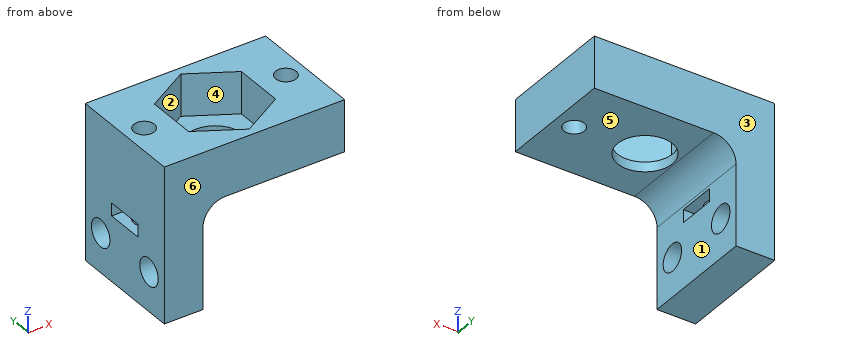
from build123d import *

# Parameters (mm, degrees)
BOSS_EXTRUDE1_DEPTH = 18
CUT_EXTRUDE1_DEPTH  = 6.5
SKETCH4_R           = 1.6
CUT_EXTRUDE2_DEPTH  = 17
SKETCH5_W           = 2
SKETCH5_H           = 6
CUT_EXTRUDE3_DEPTH  = 6
SKETCH6_R           = 4.25
CUT_EXTRUDE4_DEPTH  = 6
FILLET1_R           = 3.5
SKETCH7_R           = 2.1
CUT_EXTRUDE5_DEPTH  = 6


with BuildPart() as part:
    # Sketch1 → Boss-Extrude1 (new body)
    with BuildSketch(Plane(origin=(0, 0, 0), x_dir=(1, 0, 0), z_dir=(0, 1, 0))):
        Polygon((0, 24.076190476), (0, 0), (28, 0), (28, 8), (6, 8), (6, 24.076190476), align=None)
    extrude(amount=BOSS_EXTRUDE1_DEPTH)

    # Sketch3 → Cut-Extrude1 (cut)
    with BuildSketch(Plane.XY):
        Polygon((20.75, 5.102885683), (20.75, 12.897114317), (14, 16.794228634), (7.25, 12.897114317), (7.25, 5.102885683), (14, 1.205771366), align=None)
    extrude(amount=-CUT_EXTRUDE1_DEPTH, mode=Mode.SUBTRACT)

    # Sketch4 → Cut-Extrude2 (cut)
    with BuildSketch(Plane.XY):
        with Locations((25, 9)):
            Circle(SKETCH4_R)
        with Locations((3, 9)):
            Circle(SKETCH4_R)
    extrude(amount=-CUT_EXTRUDE2_DEPTH, mode=Mode.SUBTRACT)

    # Sketch5 → Cut-Extrude3 (cut)
    with BuildSketch(Plane.ZY):
        with Locations((-13, 9)):
            Rectangle(SKETCH5_W, SKETCH5_H)
    extrude(amount=-CUT_EXTRUDE3_DEPTH, mode=Mode.SUBTRACT)

    # Sketch6 → Cut-Extrude4 (cut)
    with BuildSketch(Plane.XY.offset(-6.5)):
        with Locations((14, 9)):
            Circle(SKETCH6_R)
    extrude(amount=-CUT_EXTRUDE4_DEPTH, mode=Mode.SUBTRACT)

    # Fillet1
    fillet1_edges = [part.edges().sort_by_distance(p)[0] for p in [
        (6, 9, -8),
    ]]
    fillet(fillet1_edges, radius=FILLET1_R)

    # Sketch7 → Cut-Extrude5 (cut)
    with BuildSketch(Plane(origin=(6, 0, 0), x_dir=(0, 0, -1), z_dir=(1, 0, 0))):
        with Locations((18, 14.5)):
            Circle(SKETCH7_R)
        with Locations(Location((18, 3.5, 0), (0, 0, 180))):
            Circle(SKETCH7_R)
    extrude(amount=-CUT_EXTRUDE5_DEPTH, mode=Mode.SUBTRACT)


solid = part.part
Build history of the part. All positions in model axes, mm. Face numbers are marked on the shaded views. A direction names the side the tool comes from. Coordinates: 2 decimals unless noted, no trailing zeros. Order: outer loops, then holes, each group sorted by start corner. A loop starts at its lowest first (then second) coordinate and runs counter-clockwise, first axis right, second up. Notation, with made-up numbers: (-37, 78) -> (-5, 78) arc R16 ccw to (-5, 108) -> close; hole circle Ø8 at (46, -35.75). An arc over 180 degrees is marked (long way). One line per item, written item: value.
(1) Slice it at C-C, the plane z = -13.5. List the corners of the cut face in (x, y), plus the area to 3 significant figures.
Checked values:
outline: (0, 0) -> (6, 0) -> (6, 6) -> (0, 6) -> close; (0, 12) -> (6, 12) -> (6, 18) -> (0, 18) -> close
area: 72.0 mm2
(2) Tool access for the marked faces 1, 2 and 3: list every direction of +Z, -Z, +X, -X, +Y, -Y with a clear straight run to the whole face (end or side of a thin tool).
Checked values:
face 1: -Z, +X, +Y, -Y
face 2: +Z
face 3: +Z, -Z, +X, -X, +Y
(3) Slice it at B-B, the plane y = 9. Count the separate pieces of the cut face and the enclosed holes in it, plus the area to 3 significant figures.
Checked values:
separate pieces: 5
enclosed holes: 0
area: 137 mm2
(4) Probe line 1 (Y direction, x = 4.55, z = -18); line 2 (Y direction, x = 3, z = -9.25); line 3 (X direction, y = 11.5, z = -1.5). List the from-to ranges inside material, lowest first. Write a range as [from, to].
Checked values:
line 1: [0, 1.4], [5.6, 12.4], [16.6, 18]
line 2: [0, 7.4], [10.6, 18]
line 3: [0, 7.25], [20.75, 28]
(5) Slice it at D-D, the plane z = -18. List the corners of the cut face in (x, y).
Checked values:
outline: (0, 0) -> (6, 0) -> (6, 1.4) -> (0, 1.4) -> close; (0, 5.6) -> (6, 5.6) -> (6, 12.4) -> (0, 12.4) -> close; (0, 16.6) -> (6, 16.6) -> (6, 18) -> (0, 18) -> close
(6) Drop flat-ended pins along their axis: pin 1 Ø7 at (x, y) = (14, 6.5) entering from +Z; pin 2 Ø9 at (x, y) = (19, 6.5) entering from -Z; pin 3 Ø2 at (y, z) = (5.5, -19) entering from +X; pin 4 Ø4 at (y, z) = (14.5, -18) entering from +X. Give the stop position or say it passes through.
Checked values:
pin 1: z = -6.5
pin 2: z = -8
pin 3: x = 6
pin 4: through
(7) Slice it at A-A, the plane x = 25. List the corners of the cut face in (y, z), plus the area to 3 significant figures.
Checked values:
outline: (0, -8) -> (7.4, -8) -> (7.4, 0) -> (0, 0) -> close; (10.6, -8) -> (18, -8) -> (18, 0) -> (10.6, 0) -> close
area: 118 mm2
(8) Mould opens along Y. For the marked faces 4, 5 and 6 say: pulls with the +Y half, pulls with the -Y half, needs draft (parallel to the pull), parting line crosses it, or undercut.
Checked values:
face 4: undercut
face 5: needs draft
face 6: pulls with the -Y half
